from build123d import *

# Parameters (mm, degrees)
F0_R      = 2.15
F1_DEPTH  = 3
F2_W      = 40
F2_H      = 3
F3_DEPTH  = 20
F5_DEPTH  = 4
F7_START  = -12
F7_DEPTH  = 3
F8_START  = -25
F8_DEPTH  = 3
F10_DEPTH = 1


with BuildPart() as f1:
    # F0 (on Top) → F1 (new body)
    with BuildSketch(Plane.XY):
        Polygon((-8, 4.2815308196), (-8, -7.7184691804), (8, -7.7184691804), (8, 4.2815308196), (8, 23.7919500181), (-8, 23.7919500181), align=None)
        with BuildLine():
            ThreePointArc((-1.55, 18.7919500181), (0, 20.3419500181), (1.55, 18.7919500181))
            Line((1.55, 18.7919500181), (1.55, 2.2815308196))
            ThreePointArc((1.55, 2.2815308196), (0, 0.7315308196), (-1.55, 2.2815308196))
            Line((-1.55, 2.2815308196), (-1.55, 18.7919500181))
        make_face(mode=Mode.SUBTRACT)
        with BuildLine():
            ThreePointArc((-8, 4.2815308196), (-11.5147186258, -4.2037505546), (-20, -7.7184691804))
            Line((-20, -7.7184691804), (-8, -7.7184691804))
            Line((-8, -7.7184691804), (-8, 4.2815308196))
        make_face()
        with BuildLine():
            Line((8, 4.2815308196), (8, -7.7184691804))
            Line((8, -7.7184691804), (20, -7.7184691804))
            ThreePointArc((20, -7.7184691804), (11.5147186258, -4.2037505546), (8, 4.2815308196))
        make_face()
        Polygon((-8, -7.7184691804), (-20, -7.7184691804), (-20, -30.7184691804), (20, -30.7184691804), (20, -7.7184691804), (8, -7.7184691804), align=None)
        with Locations((-9.6621733536, -19.2184691804)):
            Circle(F0_R, mode=Mode.SUBTRACT)
        with Locations((9.6621733536, -19.2184691804)):
            Circle(F0_R, mode=Mode.SUBTRACT)
    extrude(amount=F1_DEPTH)

    # F2 (on face) → F3 (join)
    with BuildSketch(Plane.XY.offset(3)):
        with Locations((0, -9.2184691804)):
            Rectangle(F2_W, F2_H)
    extrude(amount=F3_DEPTH)

    # F4 (on face) → F5 (cut)
    with BuildSketch(Plane.XZ.offset(10.7184691804)):
        with BuildLine():
            Line((-20, 23), (-20, 11))
            ThreePointArc((-20, 11), (-11.5147186258, 14.5147186258), (-8, 23))
            Line((-8, 23), (-20, 23))
        make_face()
        with BuildLine():
            Line((20, 23), (8, 23))
            ThreePointArc((8, 23), (11.5147186258, 14.5147186258), (20, 11))
            Line((20, 11), (20, 23))
        make_face()
    extrude(amount=-F5_DEPTH, mode=Mode.SUBTRACT)

    # F6 (on face) → F7 (join)
    with BuildSketch(Plane.YZ.offset(20).offset(F7_START)):
        Polygon((23.7919500181, 3), (-7.7184691804, 23), (-7.7184691804, 11), (-7.7184691804, 3), align=None)
    extrude(amount=-F7_DEPTH)

    # F6 (on face) → F8 (join)
    with BuildSketch(Plane.YZ.offset(20).offset(F8_START)):
        Polygon((23.7919500181, 3), (-7.7184691804, 23), (-7.7184691804, 3), align=None)
    extrude(amount=-F8_DEPTH)

    # F9 (on face) → F10 (cut)
    with BuildSketch(Plane.XY.offset(3)):
        Polygon((1.2478875427, 21.9026152913), (-1.2478875427, 21.9026152913), (-2.5953908917, 20.6514410675), (-2.5953908917, 0), (-1.2478875427, -1.1958031218), (1.2478875427, -1.1958031218), (2.5953908917, 0), (2.5953908917, 20.6514410675), align=None)
        with BuildLine():
            Line((-1.55, 2.2815308196), (-1.55, 18.7919500181))
            ThreePointArc((-1.55, 18.7919500181), (0, 20.3419500181), (1.55, 18.7919500181))
            Line((1.55, 18.7919500181), (1.55, 2.2815308196))
            ThreePointArc((1.55, 2.2815308196), (0, 0.7315308196), (-1.55, 2.2815308196))
        make_face(mode=Mode.SUBTRACT)
    extrude(amount=-F10_DEPTH, mode=Mode.SUBTRACT)


solid = f1.part
Design review of the part built by this model. Coordinates are the model's own, in mm. A direction names the side the tool comes from. Coordinates: 2 decimals unless noted, no trailing zeros. Order: outer loops, then holes, each group sorted by start corner. A loop starts at its lowest first (then second) coordinate and runs counter-clockwise, first axis right, second up. Notation, with made-up numbers: M 30.5,58 L 60.5,58 A7 ccw 60.5,65 Z; hole C -13,68.25 d5. An arc over 180 degrees is marked long. Use a Markdown table: item, result.
(1) Wall thickness on probe 1 along X at (y, z) = (9, 2.25); probe 2 along X at (y, z) = (-2.5, 12.5); probe 3 along Y at (x, z) = (11, 8.5): over which ranges is each line inside the solid? List them lowest first.
Worked answers:
| item | result |
|---|---|
| probe 1 | x = -8 to -2.6, 2.6 to 8 |
| probe 2 | x = -8 to -5, 5 to 8 |
| probe 3 | y = -10.72 to -7.72 |
(2) Add section A-A (x = 0). Give the boundary of the cut face in (y, z), then the cut area to 3 significant figures.
Worked answers:
| item | result |
|---|---|
| outline | M -30.72,0 L 0.73,0 L 0.73,2 L -1.2,2 L -1.2,3 L -7.72,3 L -7.72,23 L -10.72,23 L -10.72,3 L -30.72,3 Z; M 20.34,0 L 23.79,0 L 23.79,3 L 21.9,3 L 21.9,2 L 20.34,2 Z |
| area | 161 mm2 |
(3) Add section C-C (z = 14). Give the boundary of the cut face in (x, y), then the cut area to 3 significant figures.
Worked answers:
| item | result |
|---|---|
| outline | M -12.06,-10.72 L 12.06,-10.72 L 12.06,-7.72 L 8,-7.72 L 8,6.46 L 5,6.46 L 5,-7.72 L -5,-7.72 L -5,6.46 L -8,6.46 L -8,-7.72 L -12.06,-7.72 Z |
| area | 157 mm2 |
(4) For faces 4 (the flat face through (-2, 11, 2)), 5 (the flat face through (-1.55, 10, 1)), 6 (the flat face through (-8, 4, 9)), 7 (the flat face through (-5, 1, 9)), 8 (the flat face through (8, 4, 9)), list the 3-axis set-ups (+Z, -Z, +X, -X, +Y, -Y) from which the entire face can be reached by the end or side of a thin tool; tool diameter is ignored.
Worked answers:
| item | result |
|---|---|
| face 4 | +Z |
| face 5 | +Z, -Z |
| face 6 | +Z, -X, +Y |
| face 7 | +Z, +Y |
| face 8 | +Z, +X, +Y |
(5) Add section D-D (x = -14). Give the boundary of the cut face in (y, z).
Worked answers:
| item | result |
|---|---|
| outline | M -30.72,0 L -6.11,0 L -6.11,3 L -7.72,3 L -7.72,12.61 L -10.72,12.61 L -10.72,3 L -30.72,3 Z |
(6) For P1, Ø0.6, axis at y = 14, z = 0.5, coming from the +X side; P2, Ø6, axis at x = -6.5, y = -23, coming from the +Z side; P3, Ø13, axis at x = 17, y = 1, coming from the +Z side (1 decimal); P4, Ø3.5, axis at x = 14.5, z = 9, coming from the +Y side, all flat-tipped, find the tip position at first contact; note any pin that passes through.
Worked answers:
| item | result |
|---|---|
| P1 | stops at x = 8 |
| P2 | stops at z = 3 |
| P3 | passes through |
| P4 | stops at y = -7.72 |
(7) Add section B-B (y = 3). Give the boundary of the cut face in (x, z).
Worked answers:
| item | result |
|---|---|
| outline | M -8.07,0 L -1.55,0 L -1.55,2 L -2.6,2 L -2.6,3 L -5,3 L -5,16.2 L -8,16.2 L -8,3 L -8.07,3 Z; M 1.55,0 L 8.07,0 L 8.07,3 L 8,3 L 8,16.2 L 5,16.2 L 5,3 L 2.6,3 L 2.6,2 L 1.55,2 Z |
(8) Draft analysis for pull direction X (two halves, no side actions). For faces 1 (the flat face through (1.91, -0.61, 2.51)), 2 (the flat face through (-10, -5, 3)), 3 (the cylindrical face through (-11.42, -4.11, 1.48)), state which applies: released by +X, released by -X, zero draft, split by the parting line, or undercut.
Worked answers:
| item | result |
|---|---|
| face 1 | undercut |
| face 2 | zero draft |
| face 3 | released by -X |
